Geometry: final body of the model. Coordinates: model frame, mm. Face numbers are marked on the shaded views. Give positions to 0.01 mm unless a question says otherwise; leave off trailing zeros. Loops run counter-clockwise (first coordinate to the right, second up) from the corner with the lowest first, then second, coordinate; pieces in that order, holes last. Notation, with made-up numbers: (40.5, 77.5) -> (47.5, 77.5) arc R19 cw to (47.5, 90.5) -> close; hole circle Ø4 at (-1, 42.25). An arc over 180 degrees is marked (long way). Answer in a Markdown table with one row per item. Add a question column.
1) Section query C-C (y = -2). Return the cut outline in (x, z).
2) Draft query along Z for the marked faces 1, 2, 3 and 4. Return one class per face: +Z half, -Z half, draft (parallel to the pull), parting line (faces both ways), or undercut.
3) Section query A-A (z = 0). Return the cut outline in (x, y) (3 decimals).
4) Section query B-B (z = 54). Return the cut outline in (x, y), plus the area to 3 significant figures.
5) First-contact query: P1, Ø5.5, axis at x = -9.5, z = 53.5, coming from the +Y side; P2, Ø6, axis at y = 11, z = -15, coming from the -X side; P3, Ø4, axis at x = 48.21, z = 0, coming from the -Y side; P4, Ø8, axis at x = -6, y = 28.5, coming from the +Z side. Flat tips, straight axial feed; report the tip coordinate or a pass-through.
6) Line query: line 1 (X direction, y = 1, z = 0); line 2 (Z direction, x = -6, y = 23); line 3 (Y direction, x = -12.5, z = -26.5). Output: solid intervals per line, ascending. Write a range as from..to.
7) Section query D-D (x = 22). Return the cut outline in (y, z), plus the area to 3 significant figures.
```python
from build123d import *

# Parameters (mm, degrees)
BOSS_EXTRUDE1_DEPTH = 3
SKETCH4_R           = 1.5
CUT_EXTRUDE1_DEPTH  = 3
CIRPATTERN3_COUNT   = 4
CIRPATTERN4_COUNT   = 4
SKETCH6_R           = 5.46227
CUT_EXTRUDE2_DEPTH  = 3


with BuildPart() as part:
    # Sketch2 → Revolve3 (revolve)
    with BuildSketch(Plane.XY):
        Polygon((-5.787265578, 31.851275917), (40.212734422, 31.851275917), (40.212734422, -7.148724083), (43.212734422, -7.148724083), (43.212734422, 34.851275917), (-5.787265578, 34.851275917), align=None)
    revolve(axis=Axis((-5.787265578, 31.851275917, 0), (0, 1, 0)))

    # Sketch3 → Boss-Extrude1 (add)
    with BuildSketch(Plane(origin=(0, -7.148724083, 0), x_dir=(-1, 0, 0), z_dir=(0, -1, 0))):
        with BuildLine():
            Line((64.791542072, -3.977553736), (64.791542072, 0))
            Line((64.791542072, 0), (64.791542072, 3.977553736))
            Line((64.791542072, 3.977553736), (53.923592108, 9.15937051))
            ThreePointArc((53.923592108, 9.15937051), (54.570869381, 4.6), (54.787265578, 0))
            ThreePointArc((54.787265578, 0), (54.570869381, -4.6), (53.923592108, -9.15937051))
            Line((53.923592108, -9.15937051), (64.791542072, -3.977553736))
        make_face()
    boss_extrude1 = extrude(amount=-BOSS_EXTRUDE1_DEPTH)

    # Sketch4 → Cut-Extrude1 (cut)
    with BuildSketch(Plane.XZ.offset(7.148724083)):
        with Locations((-59.787265578, 0)):
            Circle(SKETCH4_R)
    cut_extrude1 = extrude(amount=-CUT_EXTRUDE1_DEPTH, mode=Mode.SUBTRACT)

    # CirPattern3: Boss-Extrude1 ×4 about axis
    cirpattern3_axis = Axis((-5.787265578, 0, 0), (0, 1, 0))
    for i in range(1, CIRPATTERN3_COUNT):
        add(boss_extrude1.rotate(cirpattern3_axis, i * 360 / CIRPATTERN3_COUNT))

    # CirPattern4: Cut-Extrude1 ×4 about axis
    cirpattern4_axis = Axis((-5.787265578, 0, 0), (0, 1, 0))
    for i in range(1, CIRPATTERN4_COUNT):
        add(cut_extrude1.rotate(cirpattern4_axis, i * 360 / CIRPATTERN4_COUNT), mode=Mode.SUBTRACT)

    # Sketch6 → Cut-Extrude2 (cut)
    with BuildSketch(Plane(origin=(0, 34.851275917, 0), x_dir=(1, 0, 0), z_dir=(0, 1, 0))):
        with Locations((-5.787265578, 0)):
            Circle(SKETCH6_R)
    extrude(amount=-CUT_EXTRUDE2_DEPTH, mode=Mode.SUBTRACT)


solid = part.part
```
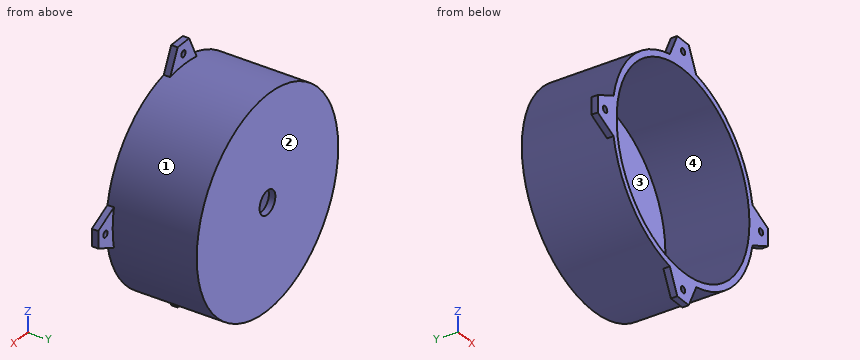
Evaluation:
| question | item | result |
|---|---|---|
| 1 | outline | circle Ø98 at (-5.79, 0); hole circle Ø92 at (-5.79, 0) |
| 2 | face 1 | parting line |
| 2 | face 2 | draft |
| 2 | face 3 | undercut |
| 2 | face 4 | undercut |
| 3 | outline | (-64.792, -7.149) -> (-61.287, -7.149) -> (-61.287, -4.149) -> (-64.792, -4.149) -> close; (-58.287, -7.149) -> (-51.787, -7.149) -> (-51.787, 31.851) -> (-11.25, 31.851) -> (-11.25, 34.851) -> (-54.787, 34.851) -> (-54.787, -4.149) -> (-58.287, -4.149) -> close; (-0.325, 31.851) -> (40.213, 31.851) -> (40.213, -7.149) -> (46.713, -7.149) -> (46.713, -4.149) -> (43.213, -4.149) -> (43.213, 34.851) -> (-0.325, 34.851) -> close; (49.713, -7.149) -> (53.217, -7.149) -> (53.217, -4.149) -> (49.713, -4.149) -> close |
| 4 | outline | (-12.15, -7.15) -> (-7.29, -7.15) -> (-7.29, -4.15) -> (-12.15, -4.15) -> close; (-4.29, -7.15) -> (0.58, -7.15) -> (0.58, -4.15) -> (-4.29, -4.15) -> close |
| 4 | area | 29.2 mm² |
| 5 | P1 | y = -4.15 |
| 5 | P2 | x = -53.3 |
| 5 | P3 | y = -7.15 |
| 5 | P4 | z = 49 |
| 6 | line 1 | -54.79..-51.79, 40.21..43.21 |
| 6 | line 2 | -49..-46, 46..49 |
| 6 | line 3 | 31.85..34.85 |
| 7 | outline | (-7.15, -40.36) -> (34.85, -40.36) -> (34.85, 40.36) -> (-7.15, 40.36) -> (-7.15, 36.66) -> (31.85, 36.66) -> (31.85, -36.66) -> (-7.15, -36.66) -> close |
| 7 | area | 531 mm² |
